Here's how the part is built. I have some questions about the finished solid (model axes, mm). A direction names the side the tool comes from. Coordinates: 2 decimals unless noted, no trailing zeros. Loops run counter-clockwise (first coordinate to the right, second up) from the corner with the lowest first, then second, coordinate; pieces in that order, holes last. Notation, with made-up numbers: M 15.5,22 L 48.5,22 A19 cw 48.5,28 Z; hole C 45.25,57 d5. An arc over 180 degrees is marked long. Use one line per item in the form item = value. Start each with the question number.
(1) Imagine slicing it at C-C, the plane y = -2. Please give me the cut outline in (x, z).
(2) Please list where these lines run through material, in increasing order: L1, parallel to Z at x = 0, y = -2.05; L2, parallel to X at y = -4.75, z = -0.5; L3, parallel to X at y = -1.75, z = 10.
(3) Will these pins go through, and if not, where does the flat tip stop? P1, Ø1.5, axis at y = -4, z = -12, coming from the -X side; P2, Ø3, axis at x = 0, z = 0, coming from the +Y side; P3, Ø1.5, axis at x = 17, y = -4, coming from the +Z side.
(4) On a 3-axis mill with a long thin cutter (end or side, diameter ignored), from which of +Z, -Z, +X, -X, +Y, -Y can I reach the whole of each face in a straight line? I mean faces 4 (the flat face through (0, -4.5, 0)), 5 (the flat face through (4, 0, 0)). Say none if no direction works.
(5) Imagine slicing it at B-B, the plane z = 0. Please give me the cut outline in (x, y), and give its area (3 significant figures).
(6) Imagine slicing it at A-A, the plane x = 0. Please give me the cut outline in (y, z), and give its area (3 significant figures).
(7) Thinking about a two-plate mould opening in X: for faces 1 (the cylindrical face through (0, -2, -2)), 2 (the flat face through (0, -6, 0)), 3 (the cylindrical face through (-2.799, -2.965, 21.317)), which applies, +X half, -X half, draft (parallel to the pull), parting line (faces both ways), or undercut?
```python
from build123d import *

# Parameters (mm, degrees)
F0_R     = 21.5
F1_DEPTH = 6
F2_R     = 2
F3_DEPTH = 4.5
F4_R     = 0.5


with BuildPart() as f1:
    # F0 (on Front) → F1 (new body)
    with BuildSketch(Plane.XZ):
        Circle(F0_R)
    extrude(amount=F1_DEPTH)

    # F2 (on face) → F3 (cut)
    with BuildSketch(Plane(origin=(0, 0, 0), x_dir=(-1, 0, 0), z_dir=(0, 1, 0))):
        Circle(F2_R)
    extrude(amount=-F3_DEPTH, mode=Mode.SUBTRACT)

    # F4
    f4_edges = [f1.edges().sort_by_distance(p)[0] for p in [
        (-21.5, 0, 0),
        (-21.5, -6, 0),
    ]]
    fillet(f4_edges, radius=F4_R)


solid = f1.part
```
Answer:
q1.outline = C 0,0 d43; hole C 0,0 d4
q2.L1 = -21.5 to -2, 2 to 21.5
q2.L2 = -21.49 to 21.49
q2.L3 = -19.03 to 19.03
q3.P1 = -18.32
q3.P2 = -4.5
q3.P3 = 14.08
q4.face_4 = +Y
q4.face_5 = +Z, -Z, +X, -X, +Y
q5.outline = M -21.5,-5.5 A0.5 ccw -21,-6 L 21,-6 A0.5 ccw 21.5,-5.5 L 21.5,-0.5 A0.5 ccw 21,0 L 2,0 L 2,-4.5 L -2,-4.5 L -2,0 L -21,0 A0.5 ccw -21.5,-0.5 Z
q5.area = 240 mm²
q6.outline = M -6,-21 A0.5 ccw -5.5,-21.5 L -0.5,-21.5 A0.5 ccw 0,-21 L 0,-2 L -4.5,-2 L -4.5,2 L 0,2 L 0,21 A0.5 ccw -0.5,21.5 L -5.5,21.5 A0.5 ccw -6,21 Z
q6.area = 240 mm²
q7.face_1 = undercut
q7.face_2 = draft
q7.face_3 = parting line
